Part model, mm, in its own coordinate system. Give positions to 0.01 mm unless a question says otherwise; leave off trailing zeros. Write each loop counter-clockwise with the first axis right and the second up, starting at its lowest first coordinate (ties: lowest second). Pieces come first, ordered by that corner, then holes. Notation, with made-up numbers: (5.25, -32.5) - (48.25, -32.5) arc R18 cw to (48.25, -7.5) - close; hole circle Ø4 at (71, 7.25). An arc over 180 degrees is marked (long way). Answer as a JSON object with one key per item and string values. Group by question number.
```python
from build123d import *

# Parameters (mm, degrees)
F0_W     = 80
F0_H     = 30
F1_DEPTH = 25
F3_D     = 8


with BuildPart() as f1:
    # F0 (on Front) → F1 (new body)
    with BuildSketch(Plane.XZ):
        Rectangle(F0_W, F0_H)
    extrude(amount=F1_DEPTH)

    # F3 (through all)
    with Locations(Plane(origin=(0, 0, -15), x_dir=(1, 0, 0), z_dir=(0, 0, -1))):
        with Locations((-32.076024, 17.399574), (-20.076024, 17.399574), (-8.076024, 17.399574), (3.923976, 17.399574), (15.923976, 17.399574), (27.923976, 17.399574), (27.923976, 7.399574), (15.923976, 7.399574), (3.923976, 7.399574), (-20.076024, 7.399574), (-32.076024, 7.399574), (-8.076024, 7.399574)):
            Hole(F3_D / 2)


solid = f1.part
```
1) Band-saw the part on D-D (y = -18.75). List the corners of the cut face in (x, z), plus the area to 3 significant figures.
2) Band-saw the part on C-C (x = -5). List the corners of the cut face in (y, z), plus the area to 3 significant figures.
3) Mould opens along X. For faces 1 (the flat face through (40, -12, 0)), 2 (the flat face through (-40, -12, 0)), 3 (the flat face through (-1, -12, -15)), 4 (the cylindrical face through (-7.209, -13.495, 0.21)) say: pulls with the +X half, pulls with the -X half, needs draft (parallel to the pull), parting line crosses it, or undercut.
4) Band-saw the part on A-A (y = -5.75). List the corners of the cut face in (x, z), plus the area to 3 significant figures.
5) Probe line 1 (Y direction, x = 16, z = -7); line 2 (Y direction, x = 17, z = 12.5). List the from-to ranges inside material, lowest first.
6) Drop a flat-ended pin along its axis: P1, Ø6.5, axis at x = 15.92, y = -17.4, coming from the +Z side. Give the stop position or say it passes through.
7) Band-saw the part on B-B (z = -5.75). State how many separate pieces and enclosed holes the cut face has, plus the area to 3 significant figures.
Verdict:
{
 "1": {"outline": "(-40, -15) - (-35.84, -15) - (-35.84, 15) - (-40, 15) - close; (-28.31, -15) - (-23.84, -15) - (-23.84, 15) - (-28.31, 15) - close; (-16.31, -15) - (-11.84, -15) - (-11.84, 15) - (-16.31, 15) - close; (-4.31, -15) - (0.16, -15) - (0.16, 15) - (-4.31, 15) - close; (7.69, -15) - (12.16, -15) - (12.16, 15) - (7.69, 15) - close; (19.69, -15) - (24.16, -15) - (24.16, 15) - (19.69, 15) - close; (31.69, -15) - (40, -15) - (40, 15) - (31.69, 15) - close", "area": "1,040 mm2"},
 "2": {"outline": "(-25, -15) - (-19.96, -15) - (-19.96, 15) - (-25, 15) - close; (-14.84, -15) - (-9.96, -15) - (-9.96, 15) - (-14.84, 15) - close; (-4.84, -15) - (0, -15) - (0, 15) - (-4.84, 15) - close", "area": "443 mm2"},
 "3": {"face 1": "pulls with the +X half", "face 2": "pulls with the -X half", "face 3": "needs draft", "face 4": "undercut"},
 "4": {"outline": "(-40, -15) - (-35.72, -15) - (-35.72, 15) - (-40, 15) - close; (-28.43, -15) - (-23.72, -15) - (-23.72, 15) - (-28.43, 15) - close; (-16.43, -15) - (-11.72, -15) - (-11.72, 15) - (-16.43, 15) - close; (-4.43, -15) - (0.28, -15) - (0.28, 15) - (-4.43, 15) - close; (7.57, -15) - (12.28, -15) - (12.28, 15) - (7.57, 15) - close; (19.57, -15) - (24.28, -15) - (24.28, 15) - (19.57, 15) - close; (31.57, -15) - (40, -15) - (40, 15) - (31.57, 15) - close", "area": "1,090 mm2"},
 "5": {"line 1": "-25 to -21.4, -13.4 to -11.4, -3.4 to 0", "line 2": "-25 to -21.25, -13.55 to -11.25, -3.55 to 0"},
 "6": {"P1": "through"},
 "7": {"separate pieces": "1", "enclosed holes": "12", "area": "1,400 mm2"}
}
